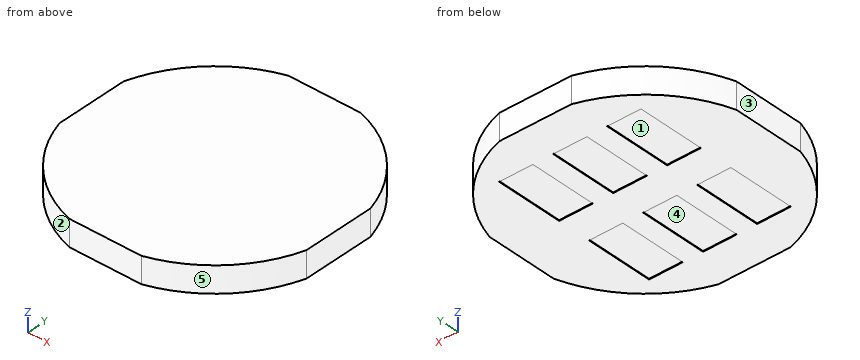
from build123d import *

# Parameters (mm, degrees)
BOSS_EXTRUDE1_DEPTH = 0.9652
SKETCH2_W           = 1.25
SKETCH2_H           = 2.5
CUT_EXTRUDE1_DEPTH  = 0.0254


with BuildPart() as part:
    # Sketch1 → Boss-Extrude1 (new body)
    with BuildSketch(Plane.XY):
        with BuildLine():
            Line((-1.3335, 4.572), (1.3335, 4.572))
            ThreePointArc((1.3335, 4.572), (3.367596045, 3.367596045), (4.572, 1.3335))
            Line((4.572, 1.3335), (4.572, -1.3335))
            ThreePointArc((4.572, -1.3335), (3.367596045, -3.367596045), (1.3335, -4.572))
            Line((1.3335, -4.572), (-1.3335, -4.572))
            ThreePointArc((-1.3335, -4.572), (-3.367596045, -3.367596045), (-4.572, -1.3335))
            Line((-4.572, -1.3335), (-4.572, 1.3335))
            ThreePointArc((-4.572, 1.3335), (-3.367596045, 3.367596045), (-1.3335, 4.572))
        make_face()
    extrude(amount=-BOSS_EXTRUDE1_DEPTH)

    # Sketch2 → Cut-Extrude1 (cut)
    with BuildSketch(Plane(origin=(0, 0, -0.9652), x_dir=(-1, 0, 0), z_dir=(0, 0, -1))):
        with Locations((-2, 1.875)):
            Rectangle(SKETCH2_W, SKETCH2_H)
        with Locations((0, 1.875)):
            Rectangle(SKETCH2_W, SKETCH2_H)
        with Locations((2, 1.875)):
            Rectangle(SKETCH2_W, SKETCH2_H)
        with Locations((-2, -1.875)):
            Rectangle(SKETCH2_W, SKETCH2_H)
        with Locations((0, -1.875)):
            Rectangle(SKETCH2_W, SKETCH2_H)
        with Locations((2, -1.875)):
            Rectangle(SKETCH2_W, SKETCH2_H)
    extrude(amount=-CUT_EXTRUDE1_DEPTH, mode=Mode.SUBTRACT)


solid = part.part
Geometry check sheet. Reference: the model listing, model coordinates, mm. Face numbers are marked on the shaded views. A direction names the side the tool comes from. Coordinates: 2 decimals unless noted, no trailing zeros. Order: outer loops, then holes, each group sorted by start corner. A loop starts at its lowest first (then second) coordinate and runs counter-clockwise, first axis right, second up. Notation, with made-up numbers: (2, 37.5) - (6, 37.5) arc R21 ccw to (6, 48.5) - close; hole circle Ø6 at (5, 47). An arc over 180 degrees is marked (long way). One line per item, written item: value.
(1) Thickness scan on probe 1 along Z at (x, y) = (-0.25, 2); probe 2 along X at (y, z) = (2.25, -0.75); probe 3 along Y at (x, z) = (4, -0.5). Record the ranges inside material, lowest first. Write a range as from..to.
Data:
probe 1: z = -0.94..0
probe 2: x = -4.2..4.2
probe 3: y = -2.58..2.58
(2) Access from +Z, -Z, +X, -X, +Y, -Y to the whole of each face (thin tool, end or side, straight path). Record for the marked faces 4 and 5.
Data:
face 4: -Z
face 5: +Z, -Z, +X, -Y
(3) Sectioned sample at D-D (x = 2). Enter the section's corners in (y, z) (3 decimals).
Data:
outline: (-4.322, -0.965) - (-3.125, -0.965) - (-3.125, -0.94) - (-0.625, -0.94) - (-0.625, -0.965) - (0.625, -0.965) - (0.625, -0.94) - (3.125, -0.94) - (3.125, -0.965) - (4.322, -0.965) - (4.322, 0) - (-4.322, 0) - close
(4) Sectioned sample at C-C (y = -2.75). Enter the section's corners in (x, z) (3 decimals), and give its area (3 significant figures).
Data:
outline: (-3.888, -0.965) - (-2.625, -0.965) - (-2.625, -0.94) - (-1.375, -0.94) - (-1.375, -0.965) - (-0.625, -0.965) - (-0.625, -0.94) - (0.625, -0.94) - (0.625, -0.965) - (1.375, -0.965) - (1.375, -0.94) - (2.625, -0.94) - (2.625, -0.965) - (3.888, -0.965) - (3.888, 0) - (-3.888, 0) - close
area: 7.41 mm^2
(5) Depth check by flat-ended pin: pin 1 Ø1 at (x, y) = (-2, -1.5) entering from -Z. Enter the tip coordinate at first touch or a pass-through.
Data:
pin 1: stops at z = -0.94
(6) Release check for a two-part mould opening along Y. For the marked faces 1, 2 and 3 record: +Y half, -Y half, draft (parallel to the pull), parting line (faces both ways), or undercut.
Data:
face 1: undercut
face 2: -Y half
face 3: draft
(7) Sectioned sample at A-A (z = -0.65). Enter the section's corners in (x, y) (1 decimal).
Data:
outline: (-4.6, -1.3) arc R4.8 ccw to (-1.3, -4.6) - (1.3, -4.6) arc R4.8 ccw to (4.6, -1.3) - (4.6, 1.3) arc R4.8 ccw to (1.3, 4.6) - (-1.3, 4.6) arc R4.8 ccw to (-4.6, 1.3) - close
(8) Sectioned sample at B-B (x = -1.5). Enter the section's corners in (y, z) (3 decimals), and give its area (3 significant figures).
Data:
outline: (-4.52, -0.965) - (-3.125, -0.965) - (-3.125, -0.94) - (-0.625, -0.94) - (-0.625, -0.965) - (0.625, -0.965) - (0.625, -0.94) - (3.125, -0.94) - (3.125, -0.965) - (4.52, -0.965) - (4.52, 0) - (-4.52, 0) - close
area: 8.60 mm^2
